Source: CAD feature listing. Evaluate the final solid. Frame: model axes, mm. Round coordinates to 2 decimals unless told otherwise and drop trailing zeros. Loops run counter-clockwise (first coordinate to the right, second up) from the corner with the lowest first, then second, coordinate; pieces in that order, holes last. Notation, with made-up numbers: M 86,28.25 L 136,28.25 A13 cw 136,45.25 Z; hole C -11,89 d2. An arc over 180 degrees is marked long. Write each question's results on one line, items separated by ' | '. Start each with the question number.
1. Section A-A on z = 4. Output: boundary loops of the cut face in (x, y).
2. Contact query for flat-ended pins moving along their axis: pin 1 Ø3 at (x, z) = (-43.5, 3.5) entering from -Y; pin 2 Ø4 at (x, y) = (-47.5, -9.5) entering from -Z; pin 3 Ø3 at (y, z) = (14.5, 4.5) entering from -X. Output: stop coordinate, or through.
3. Ray query, line 1 (Y direction, x = -47, z = 2.5); line 2 (X direction, y = 40.5, z = 3.5). Return the intervals inside material, ascending.
4. Section B-B on x = -52.5. Output: boundary loops of the cut face in (y, z), and give its area (3 significant figures).
Autodesk Inventor part; units mm, degrees
ref_plane "YZ Plane" through (0, 0, 0) normal (1, 0, 0) x (0, 1, 0)
ref_plane "XZ Plane" through (0, 0, 0) normal (0, 1, 0) x (-1, 0, 0)
ref_plane "XY Plane" through (0, 0, 0) normal (0, 0, 1) x (1, 0, 0)
sketch "Sketch1" plane through (0, 0, 0) normal (0, 0, 1) x (1, 0, 0)
  line L0 (-215, 60) -> (215, 60)
  line L1 (215, 60) -> (215, -60)
  line L2 (215, -60) -> (-215, -60)
  line L3 (-215, -60) -> (-215, 60)
  point P0 (0, 0)
  dimension "d0" = 120
  dimension "d1" = 430
  dimension "d2" = 215
  dimension "d3" = 60
extrude "Extrusion1" add sketch "Sketch1" along normal blind 6.35
sketch "Sketch2" plane through (0, 0, 6.35) normal (0, 0, 1) x (1, 0, 0)
  line L0 (215, 60) -> (-215, 60)
  line L1 (-215, 60) -> (-208.65, 60)
  line L2 (-208.65, 60) -> (-208.65, 40)
  line L3 (-208.65, 40) -> (-215, 40)
  line L4 (-215, 40) -> (-215, 60)
  line L5 (-215, 60) -> (-215, -60)
  line L6 (-215, 20) -> (-208.65, 20)
  line L7 (-208.65, 20) -> (-208.65, 0)
  line L8 (-208.65, 0) -> (-215, 0)
  line L9 (-215, 0) -> (-215, 20)
  line L10 (-215, -20) -> (-208.65, -20)
  line L11 (-208.65, -20) -> (-208.65, -40)
  line L12 (-208.65, -40) -> (-215, -40)
  line L13 (-215, -40) -> (-215, -20)
  line L14 (-215, -60) -> (-215, -55)
  line L15 (215, 60) -> (208.65, 60)
  line L16 (208.65, 60) -> (208.65, 40)
  line L17 (208.65, 40) -> (215, 40)
  line L18 (215, 40) -> (215, 60)
  line L19 (215, -60) -> (215, 60)
  line L20 (215, 20) -> (208.65, 20)
  line L21 (208.65, 20) -> (208.65, 0)
  line L22 (208.65, 0) -> (215, 0)
  line L23 (215, 0) -> (215, 20)
  line L24 (215, -20) -> (208.65, -20)
  line L25 (208.65, -20) -> (208.65, -40)
  line L26 (208.65, -40) -> (215, -40)
  line L27 (215, -40) -> (215, -20)
  line L28 (215, -60) -> (215, 60)
  line L29 (215, -60) -> (215, -55)
  point P0 (0, 0)
  point P1 (208.65, -60)
  dimension "d6" = 6.35
  dimension "d7" = 20
  dimension "d8" = 20
  dimension "d9" = 20
  dimension "d10" = 20
  dimension "d11" = 20
  dimension "d13" = 20
  dimension "d14" = 20
  dimension "d15" = 20
  dimension "d16" = 20
  dimension "d17" = 20
  dimension "d19" = 6.35
extrude "Extrusion2" cut sketch "Sketch2" against normal through all
sketch "Sketch3" plane through (0, 0, 6.35) normal (0, 0, 1) x (1, 0, 0)
  line L0 (-215, -60) -> (215, -60)
  line L1 (-65, -60) -> (5, -60)
  line L2 (5, -60) -> (5, -53.65)
  line L3 (5, -53.65) -> (-65, -53.65)
  line L4 (-65, -53.65) -> (-65, -60)
  line L5 (115, -60) -> (185, -60)
  line L6 (185, -60) -> (185, -53.65)
  line L7 (185, -53.65) -> (115, -53.65)
  line L8 (115, -53.65) -> (115, -60)
  point P0 (0, 0)
  point P1 (-268.65, -60)
  point P2 (268.65, -60)
  point P3 (185, -60)
  dimension "d22" = 70
  dimension "d23" = 70
  dimension "d25" = 110
  dimension "d26" = 6.35
  dimension "d27" = 6.35
  dimension "d30" = 150
extrude "Extrusion3" cut sketch "Sketch3" against normal through all
sketch "Sketch4" plane through (0, 0, 6.35) normal (0, 0, 1) x (1, 0, 0)
  line L0 (208.65, 60) -> (-208.65, 60)
  line L1 (208.65, 60) -> (215, 60)
  line L2 (215, 60) -> (215, -60)
  line L3 (215, -60) -> (208.65, -60)
  line L4 (208.65, -60) -> (208.65, 60)
  line L5 (185, -53.65) -> (185, -60) construction
  line L6 (185, -60) -> (215, -60) construction
  line L7 (215, -60) -> (215, -40) construction
  line L8 (215, -40) -> (208.65, -40) construction
  line L9 (208.65, -40) -> (208.65, -20) construction
  line L10 (208.65, -20) -> (215, -20) construction
  line L11 (215, -20) -> (215, 0) construction
  line L12 (215, 0) -> (208.65, 0) construction
  line L13 (208.65, 0) -> (208.65, 20) construction
  line L14 (208.65, 20) -> (215, 20) construction
  line L15 (215, 20) -> (215, 40) construction
  line L16 (215, 40) -> (208.65, 40) construction
  line L17 (208.65, 40) -> (208.65, 60) construction
  line L18 (208.65, 60) -> (-208.65, 60)
  line L19 (-208.65, 60) -> (-208.65, 40)
  line L20 (-208.65, 40) -> (-215, 40)
  line L21 (-215, 40) -> (-215, 20)
  line L22 (-215, 20) -> (-208.65, 20)
  line L23 (-208.65, 20) -> (-208.65, 0)
  line L24 (-208.65, 0) -> (-215, 0)
  line L25 (-215, 0) -> (-215, -20)
  line L26 (-215, -20) -> (-208.65, -20)
  line L27 (-208.65, -20) -> (-208.65, -40)
  line L28 (-208.65, -40) -> (-215, -40)
  line L29 (-215, -40) -> (-215, -60)
  line L30 (-215, -60) -> (-65, -60)
  line L31 (-65, -60) -> (-65, -53.65)
  line L32 (-65, -53.65) -> (5, -53.65)
  line L33 (5, -53.65) -> (5, -60)
  line L34 (5, -60) -> (115, -60)
  line L35 (115, -60) -> (115, -53.65)
  line L36 (115, -53.65) -> (185, -53.65) construction
  point P0 (0, 0)
  point P1 (211.825, -60)
extrude "Extrusion4" cut sketch "Sketch4" against normal through all
equation "\"d10\" = d8"
equation "\"d27\" = d26"
properties part number "2202_Housing Side_V1" material "Wood (Birch)"
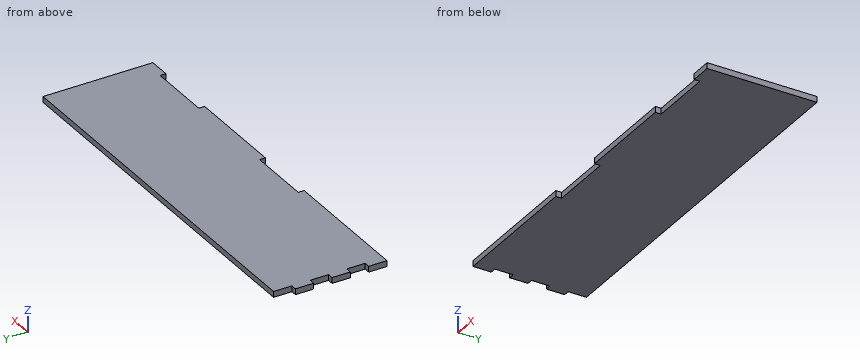
Taken from the geometry:
1) outline: M -215,-60 L -65,-60 L -65,-53.65 L 5,-53.65 L 5,-60 L 115,-60 L 115,-53.65 L 185,-53.65 L 185,-60 L 208.65,-60 L 208.65,60 L -208.65,60 L -208.65,40 L -215,40 L -215,20 L -208.65,20 L -208.65,0 L -215,0 L -215,-20 L -208.65,-20 L -208.65,-40 L -215,-40 Z
2) pin 1: y = -53.65 | pin 2: z = 0 | pin 3: x = -208.65
3) line 1: -53.65 to 60 | line 2: -208.65 to 208.65
4) outline: M -53.65,0 L 60,0 L 60,6.35 L -53.65,6.35 Z | area: 722 mm^2
